```python
from build123d import *

# Parameters (mm, degrees)
SKETCH_1_W          = 206
SKETCH_1_H          = 176
EXTRUDE_1_DEPTH     = 4.5
CUT_EXTRUDE_1_REACH = 272.984
SKETCH_2_R          = 2
CUT_EXTRUDE_2_REACH = 272.984
SKETCH_3_R          = 2.6
SKETCH_3_R_2        = 1.6


with BuildPart() as part:
    # 草图1 → 凸台-拉伸1 (new body)
    with BuildSketch(Plane.XY):
        with Locations((103, 88)):
            Rectangle(SKETCH_1_W, SKETCH_1_H)
    extrude(amount=EXTRUDE_1_DEPTH)

    # 草图2 → 切除-拉伸1 (cut, up to next)
    with BuildSketch(Plane.XY.offset(4.5), mode=Mode.PRIVATE) as cut_extrude_1_sk1:
        with Locations((12.75, 152)):
            Circle(SKETCH_2_R)
    cut_extrude_1_tool1 = extrude(cut_extrude_1_sk1.sketch, amount=-CUT_EXTRUDE_1_REACH, mode=Mode.PRIVATE) & part.part
    # 草图2 → 切除-拉伸1 (cut, up to next)
    with BuildSketch(Plane.XY.offset(4.5), mode=Mode.PRIVATE) as cut_extrude_1_sk2:
        with Locations((12.75, 130)):
            Circle(SKETCH_2_R)
    cut_extrude_1_tool2 = extrude(cut_extrude_1_sk2.sketch, amount=-CUT_EXTRUDE_1_REACH, mode=Mode.PRIVATE) & part.part
    # 草图2 → 切除-拉伸1 (cut, up to next)
    with BuildSketch(Plane.XY.offset(4.5), mode=Mode.PRIVATE) as cut_extrude_1_sk3:
        with Locations((12.75, 42)):
            Circle(SKETCH_2_R)
    cut_extrude_1_tool3 = extrude(cut_extrude_1_sk3.sketch, amount=-CUT_EXTRUDE_1_REACH, mode=Mode.PRIVATE) & part.part
    # 草图2 → 切除-拉伸1 (cut, up to next)
    with BuildSketch(Plane.XY.offset(4.5), mode=Mode.PRIVATE) as cut_extrude_1_sk4:
        with Locations((12.75, 20)):
            Circle(SKETCH_2_R)
    cut_extrude_1_tool4 = extrude(cut_extrude_1_sk4.sketch, amount=-CUT_EXTRUDE_1_REACH, mode=Mode.PRIVATE) & part.part
    # 草图2 → 切除-拉伸1 (cut, up to next)
    with BuildSketch(Plane.XY.offset(4.5), mode=Mode.PRIVATE) as cut_extrude_1_sk5:
        with Locations(Location((193.25, 20, 0), (0, 0, 180))):
            Circle(SKETCH_2_R)
    cut_extrude_1_tool5 = extrude(cut_extrude_1_sk5.sketch, amount=-CUT_EXTRUDE_1_REACH, mode=Mode.PRIVATE) & part.part
    # 草图2 → 切除-拉伸1 (cut, up to next)
    with BuildSketch(Plane.XY.offset(4.5), mode=Mode.PRIVATE) as cut_extrude_1_sk6:
        with Locations(Location((193.25, 42, 0), (0, 0, 180))):
            Circle(SKETCH_2_R)
    cut_extrude_1_tool6 = extrude(cut_extrude_1_sk6.sketch, amount=-CUT_EXTRUDE_1_REACH, mode=Mode.PRIVATE) & part.part
    # 草图2 → 切除-拉伸1 (cut, up to next)
    with BuildSketch(Plane.XY.offset(4.5), mode=Mode.PRIVATE) as cut_extrude_1_sk7:
        with Locations(Location((193.25, 130, 0), (0, 0, 180))):
            Circle(SKETCH_2_R)
    cut_extrude_1_tool7 = extrude(cut_extrude_1_sk7.sketch, amount=-CUT_EXTRUDE_1_REACH, mode=Mode.PRIVATE) & part.part
    # 草图2 → 切除-拉伸1 (cut, up to next)
    with BuildSketch(Plane.XY.offset(4.5), mode=Mode.PRIVATE) as cut_extrude_1_sk8:
        with Locations(Location((193.25, 152, 0), (0, 0, 180))):
            Circle(SKETCH_2_R)
    cut_extrude_1_tool8 = extrude(cut_extrude_1_sk8.sketch, amount=-CUT_EXTRUDE_1_REACH, mode=Mode.PRIVATE) & part.part
    add(cut_extrude_1_tool1.solids().sort_by_distance((12.75, 152, 4.5))[0], mode=Mode.SUBTRACT)
    add(cut_extrude_1_tool2.solids().sort_by_distance((12.75, 130, 4.5))[0], mode=Mode.SUBTRACT)
    add(cut_extrude_1_tool3.solids().sort_by_distance((12.75, 42, 4.5))[0], mode=Mode.SUBTRACT)
    add(cut_extrude_1_tool4.solids().sort_by_distance((12.75, 20, 4.5))[0], mode=Mode.SUBTRACT)
    add(cut_extrude_1_tool5.solids().sort_by_distance((193.25, 20, 4.5))[0], mode=Mode.SUBTRACT)
    add(cut_extrude_1_tool6.solids().sort_by_distance((193.25, 42, 4.5))[0], mode=Mode.SUBTRACT)
    add(cut_extrude_1_tool7.solids().sort_by_distance((193.25, 130, 4.5))[0], mode=Mode.SUBTRACT)
    add(cut_extrude_1_tool8.solids().sort_by_distance((193.25, 152, 4.5))[0], mode=Mode.SUBTRACT)

    # 草图3 → 切除-拉伸2 (cut, up to next)
    with BuildSketch(Plane.XY.offset(4.5), mode=Mode.PRIVATE) as cut_extrude_2_sk1:
        with Locations((31, 113)):
            Circle(SKETCH_3_R)
    cut_extrude_2_tool1 = extrude(cut_extrude_2_sk1.sketch, amount=-CUT_EXTRUDE_2_REACH, mode=Mode.PRIVATE) & part.part
    # 草图3 → 切除-拉伸2 (cut, up to next)
    with BuildSketch(Plane.XY.offset(4.5), mode=Mode.PRIVATE) as cut_extrude_2_sk2:
        with Locations((31, 62.5)):
            Circle(SKETCH_3_R)
    cut_extrude_2_tool2 = extrude(cut_extrude_2_sk2.sketch, amount=-CUT_EXTRUDE_2_REACH, mode=Mode.PRIVATE) & part.part
    # 草图3 → 切除-拉伸2 (cut, up to next)
    with BuildSketch(Plane.XY.offset(4.5), mode=Mode.PRIVATE) as cut_extrude_2_sk3:
        with Locations((31, 12)):
            Circle(SKETCH_3_R)
    cut_extrude_2_tool3 = extrude(cut_extrude_2_sk3.sketch, amount=-CUT_EXTRUDE_2_REACH, mode=Mode.PRIVATE) & part.part
    # 草图3 → 切除-拉伸2 (cut, up to next)
    with BuildSketch(Plane.XY.offset(4.5), mode=Mode.PRIVATE) as cut_extrude_2_sk4:
        with Locations((175, 12)):
            Circle(SKETCH_3_R)
    cut_extrude_2_tool4 = extrude(cut_extrude_2_sk4.sketch, amount=-CUT_EXTRUDE_2_REACH, mode=Mode.PRIVATE) & part.part
    # 草图3 → 切除-拉伸2 (cut, up to next)
    with BuildSketch(Plane.XY.offset(4.5), mode=Mode.PRIVATE) as cut_extrude_2_sk5:
        with Locations((175, 62.5)):
            Circle(SKETCH_3_R)
    cut_extrude_2_tool5 = extrude(cut_extrude_2_sk5.sketch, amount=-CUT_EXTRUDE_2_REACH, mode=Mode.PRIVATE) & part.part
    # 草图3 → 切除-拉伸2 (cut, up to next)
    with BuildSketch(Plane.XY.offset(4.5), mode=Mode.PRIVATE) as cut_extrude_2_sk6:
        with Locations((175, 113)):
            Circle(SKETCH_3_R)
    cut_extrude_2_tool6 = extrude(cut_extrude_2_sk6.sketch, amount=-CUT_EXTRUDE_2_REACH, mode=Mode.PRIVATE) & part.part
    # 草图3 → 切除-拉伸2 (cut, up to next)
    with BuildSketch(Plane.XY.offset(4.5), mode=Mode.PRIVATE) as cut_extrude_2_sk7:
        with Locations((103, 62.5)):
            Circle(SKETCH_3_R_2)
    cut_extrude_2_tool7 = extrude(cut_extrude_2_sk7.sketch, amount=-CUT_EXTRUDE_2_REACH, mode=Mode.PRIVATE) & part.part
    # 草图3 → 切除-拉伸2 (cut, up to next)
    with BuildSketch(Plane.XY.offset(4.5), mode=Mode.PRIVATE) as cut_extrude_2_sk8:
        with BuildLine():
            Line((167, 65), (112, 65))
            ThreePointArc((112, 65), (108.464466094, 66.464466094), (107, 70))
            Line((107, 70), (107, 105))
            ThreePointArc((107, 105), (108.464466094, 108.535533906), (112, 110))
            Line((112, 110), (167, 110))
            ThreePointArc((167, 110), (170.535533906, 108.535533906), (172, 105))
            Line((172, 105), (172, 70))
            ThreePointArc((172, 70), (170.535533906, 66.464466094), (167, 65))
        make_face()
    cut_extrude_2_tool8 = extrude(cut_extrude_2_sk8.sketch, amount=-CUT_EXTRUDE_2_REACH, mode=Mode.PRIVATE) & part.part
    # 草图3 → 切除-拉伸2 (cut, up to next)
    with BuildSketch(Plane.XY.offset(4.5), mode=Mode.PRIVATE) as cut_extrude_2_sk9:
        with BuildLine():
            Line((39, 110), (94, 110))
            ThreePointArc((94, 110), (97.535533906, 108.535533906), (99, 105))
            Line((99, 105), (99, 70))
            ThreePointArc((99, 70), (97.535533906, 66.464466094), (94, 65))
            Line((94, 65), (39, 65))
            ThreePointArc((39, 65), (35.464466094, 66.464466094), (34, 70))
            Line((34, 70), (34, 105))
            ThreePointArc((34, 105), (35.464466094, 108.535533906), (39, 110))
        make_face()
    cut_extrude_2_tool9 = extrude(cut_extrude_2_sk9.sketch, amount=-CUT_EXTRUDE_2_REACH, mode=Mode.PRIVATE) & part.part
    add(cut_extrude_2_tool1.solids().sort_by_distance((31, 113, 4.5))[0], mode=Mode.SUBTRACT)
    add(cut_extrude_2_tool2.solids().sort_by_distance((31, 62.5, 4.5))[0], mode=Mode.SUBTRACT)
    add(cut_extrude_2_tool3.solids().sort_by_distance((31, 12, 4.5))[0], mode=Mode.SUBTRACT)
    add(cut_extrude_2_tool4.solids().sort_by_distance((175, 12, 4.5))[0], mode=Mode.SUBTRACT)
    add(cut_extrude_2_tool5.solids().sort_by_distance((175, 62.5, 4.5))[0], mode=Mode.SUBTRACT)
    add(cut_extrude_2_tool6.solids().sort_by_distance((175, 113, 4.5))[0], mode=Mode.SUBTRACT)
    add(cut_extrude_2_tool7.solids().sort_by_distance((103, 62.5, 4.5))[0], mode=Mode.SUBTRACT)
    add(cut_extrude_2_tool8.solids().sort_by_distance((139.5, 87.5, 4.5))[0], mode=Mode.SUBTRACT)
    add(cut_extrude_2_tool9.solids().sort_by_distance((66.5, 87.5, 4.5))[0], mode=Mode.SUBTRACT)


solid = part.part
```
Read the model definition and answer for the solid it produces. Units are mm, in the model's axes. A direction names the side the tool comes from. Coordinates: 2 decimals unless noted, no trailing zeros. Loops run counter-clockwise (first coordinate to the right, second up) from the corner with the lowest first, then second, coordinate; pieces in that order, holes last. Notation, with made-up numbers: (69, 22.5) -> (112, 22.5) arc R32 ccw to (112, 54.5) -> close; hole circle Ø11 at (30, 80.5). An arc over 180 degrees is marked (long way). Return JSON: item names as keys, results as strings.
Item 1: For a pull along Y with two mould halves and no side action, classify faces 3 (the flat face through (0, 87, 2)), 4 (the cylindrical face through (35, 108, 2)), 5 (the cylindrical face through (171, 67, 2)), 6 (the flat face through (102, 0, 2)) as +Y half, -Y half, draft (parallel to the pull), parting line (faces both ways), or undercut.
Answers:
{"face 3": "draft", "face 4": "undercut", "face 5": "undercut", "face 6": "-Y half"}
Item 2: Find section D-D (z = 1.7). Count the separate pieces of the cut face and the enclosed holes in it, plus the area to 3 significant figures.
Answers:
{"separate pieces": "1", "enclosed holes": "17", "area": "30,200 mm2"}
Item 3: Find section B-B (x = 86). Determine the outline of the cut face in (y, z).
Answers:
{"outline": "(0, 0) -> (65, 0) -> (65, 4.5) -> (0, 4.5) -> close; (110, 0) -> (176, 0) -> (176, 4.5) -> (110, 4.5) -> close"}
Item 4: For faces 1 (the flat face through (206, 87, 2)), 2 (the flat face through (34, 87, 2)), determine the directions among +Z, -Z, +X, -X, +Y, -Y from which every point of the face is accessible in a straight line to the end or side of a thin tool.
Answers:
{"face 1": "+Z, -Z, +X, +Y, -Y", "face 2": "+Z, -Z"}
Item 5: Find section A-A (y = 97). Determine the outline of the cut face in (x, z), plus the area to 3 significant figures.
Answers:
{"outline": "(0, 0) -> (34, 0) -> (34, 4.5) -> (0, 4.5) -> close; (99, 0) -> (107, 0) -> (107, 4.5) -> (99, 4.5) -> close; (172, 0) -> (206, 0) -> (206, 4.5) -> (172, 4.5) -> close", "area": "342 mm2"}
Item 6: Find the intervals of material crossed by probe 1 along X at (y, z) = (100.5, 2.15); probe 2 along X at (y, z) = (152, 1.3); probe 3 along Y at (x, z) = (175, 1.25), in increasing order.
Answers:
{"probe 1": "x = 0 to 34, 99 to 107, 172 to 206", "probe 2": "x = 0 to 10.75, 14.75 to 191.25, 195.25 to 206", "probe 3": "y = 0 to 9.4, 14.6 to 59.9, 65.1 to 110.4, 115.6 to 176"}
Item 7: Find section C-C (x = 175). Determine the outline of the cut face in (y, z), plus the area to 3 significant figures.
Answers:
{"outline": "(0, 0) -> (9.4, 0) -> (9.4, 4.5) -> (0, 4.5) -> close; (14.6, 0) -> (59.9, 0) -> (59.9, 4.5) -> (14.6, 4.5) -> close; (65.1, 0) -> (110.4, 0) -> (110.4, 4.5) -> (65.1, 4.5) -> close; (115.6, 0) -> (176, 0) -> (176, 4.5) -> (115.6, 4.5) -> close", "area": "722 mm2"}
